Here's the drawing with two shaded views (mm, measured from the low corner). I have some questions. Round coordinates to 2 decimals unless told otherwise and drop trailing zeros. Write each loop counter-clockwise with the first axis right and the second up, starting at its lowest first coordinate (ties: lowest second). Pieces come first, ordered by that corner, then holes. Notation, with made-up numbers: (37, 75.25) -> (86, 75.25) arc R18 ccw to (86, 95.25) -> close; hole circle Ø7 at (3.25, 87). An arc over 180 degrees is marked (long way). Use CSV: the item, a comma, the result in double quotes.
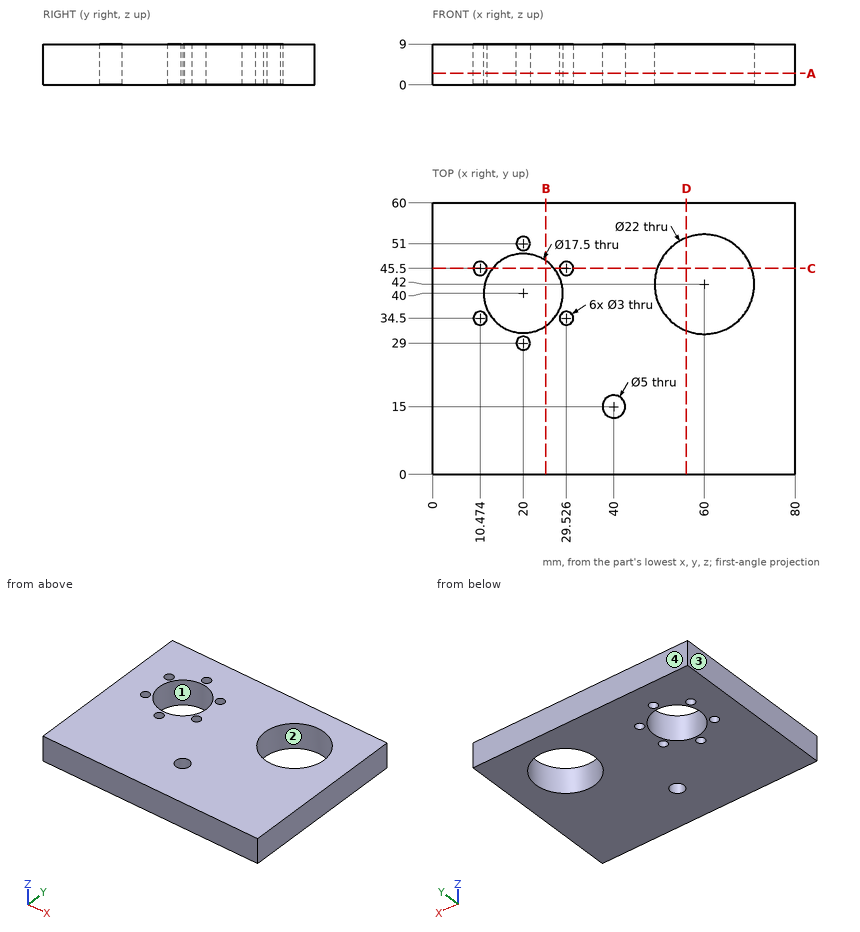
Q1. Suppose I cut it at A-A (z = 2.5). Count the separate pieces of the cut face and the enclosed holes in it, and give its area (3 significant figures).
Resolved:
separate pieces,"1"
enclosed holes,"9"
area,"4,120 mm^2"
Q2. If we mould it in two halves opening along X, with no side actions, what happens to the marked faces 1, 2, 3 and 4? For each: released by +X, released by -X, zero draft, split by the parting line, or undercut.
Resolved:
face 1,"undercut"
face 2,"undercut"
face 3,"released by -X"
face 4,"zero draft"
Q3. Suppose I cut it at D-D (x = 56). Write out the boundary of the cut face in (y, z).
Resolved:
outline,"(0, 0) -> (31.75, 0) -> (31.75, 9) -> (0, 9) -> close; (52.25, 0) -> (60, 0) -> (60, 9) -> (52.25, 9) -> close"
Q4. Suppose I cut it at C-C (y = 45.5). Write out the boundary of the cut face in (x, z) (1 decimal).
Resolved:
outline,"(0, 0) -> (9, 0) -> (9, 9) -> (0, 9) -> close; (12, 0) -> (13.2, 0) -> (13.2, 9) -> (12, 9) -> close; (26.8, 0) -> (28, 0) -> (28, 9) -> (26.8, 9) -> close; (31, 0) -> (49.6, 0) -> (49.6, 9) -> (31, 9) -> close; (70.4, 0) -> (80, 0) -> (80, 9) -> (70.4, 9) -> close"
Q5. Will this pin go through, and if not, where does the flat tip stop? P1, Ø2, axis at x = 25.5, z = 6.5, coming from the -Y side.
Resolved:
P1,"stops at y = 0"
Q6. Suppose I cut it at B-B (x = 25). Write out the boundary of the cut face in (y, z), and give its area (3 significant figures).
Resolved:
outline,"(0, 0) -> (32.82, 0) -> (32.82, 9) -> (0, 9) -> close; (47.18, 0) -> (60, 0) -> (60, 9) -> (47.18, 9) -> close"
area,"411 mm^2"
Q7. Please list where these lines run through material, in increasing order: probe 1 along Y at (x, z) = (20, 3); probe 2 along X at (y, z) = (33.5, 2.25) (1 decimal); probe 3 along X at (y, z) = (32.5, 3.75) (1 decimal).
Resolved:
probe 1,"y = 0 to 27.5, 30.5 to 31.25, 48.75 to 49.5, 52.5 to 60"
probe 2,"x = 0 to 9.4, 11.6 to 14.1, 25.9 to 28.4, 30.6 to 53, 67 to 80"
probe 3,"x = 0 to 15.5, 24.5 to 54.5, 65.5 to 80"
